from build123d import *

# Parameters (mm, degrees)
SKETCH1_R               = 15
BOSS_EXTRUDE1_DEPTH     = 27
SKETCH2_R               = 19.07
BOSS_EXTRUDE2_DEPTH     = 1.7
CUT_EXTRUDE1_DEPTH      = 23.4
SKETCH4_R               = 4
CUT_EXTRUDE2_DEPTH      = 5.3
SKETCH5_R               = 2.4
BOSS_EXTRUDE3_DEPTH     = 7
FILLET1_R               = 1
CUT_EXTRUDE3_DEPTH      = 44.397347845
CUT_EXTRUDE3_DEPTH_BACK = 44.397347845
SKETCH6_R               = 1.5


with BuildPart() as part:
    # Sketch1 → Boss-Extrude1 (new body)
    with BuildSketch(Plane(origin=(0, 0, 0), x_dir=(1, 0, 0), z_dir=(0, 1, 0))):
        with Locations(Location((0, 0, 0), (0, 0, 270))):
            Circle(SKETCH1_R)
    extrude(amount=BOSS_EXTRUDE1_DEPTH)

    # Sketch2 → Boss-Extrude2 (add)
    with BuildSketch(Plane.XZ):
        with Locations(Location((0, 0, 0), (0, 0, 270))):
            Circle(SKETCH2_R)
    extrude(amount=BOSS_EXTRUDE2_DEPTH)

    # Sketch3 → Cut-Extrude1 (cut)
    with BuildSketch(Plane.XZ.offset(1.7)):
        Polygon((-2.800148806, 4.85), (-5.600297611, 0), (-2.800148806, -4.85), (2.800148806, -4.85), (5.600297611, 0), (2.800148806, 4.85), align=None)
    extrude(amount=-CUT_EXTRUDE1_DEPTH, mode=Mode.SUBTRACT)

    # Sketch4 → Cut-Extrude2 (cut)
    with BuildSketch(Plane.XZ.offset(-21.7)):
        with Locations(Location((0, 0, 0), (0, 0, 270))):
            Circle(SKETCH4_R)
    extrude(amount=-CUT_EXTRUDE2_DEPTH, mode=Mode.SUBTRACT)

    # Sketch5 → Boss-Extrude3 (add)
    with BuildSketch(Plane(origin=(0, 27, 0), x_dir=(1, 0, 0), z_dir=(0, 1, 0))):
        with Locations(Location((-10, 0, 0), (0, 0, 270))):
            Circle(SKETCH5_R)
        with Locations(Location((10, 0, 0), (0, 0, 270))):
            Circle(SKETCH5_R)
    extrude(amount=BOSS_EXTRUDE3_DEPTH)

    # Fillet1
    fillet1_edges = [part.edges().sort_by_distance(p)[0] for p in [
        (-10, 34, -2.4),
        (10, 34, -2.4),
    ]]
    fillet(fillet1_edges, radius=FILLET1_R)

    # Sketch6 → Cut-Extrude3 (cut, two sides: drawn at the far end of the back side and taken through both)
    with BuildSketch(Plane.XY.offset(-CUT_EXTRUDE3_DEPTH_BACK)):
        with Locations(Location((0, 3, 0), (0, 0, 90))):
            Circle(SKETCH6_R)
    extrude(amount=CUT_EXTRUDE3_DEPTH + CUT_EXTRUDE3_DEPTH_BACK, mode=Mode.SUBTRACT)


solid = part.part
The listing builds one solid part. Answer for the finished solid, in the listing's coordinates (mm). A direction names the side the tool comes from. Coordinates: 2 decimals unless noted, no trailing zeros. Write each loop counter-clockwise with the first axis right and the second up, starting at its lowest first coordinate (ties: lowest second). Pieces come first, ordered by that corner, then holes. Notation, with made-up numbers: (67.5, -4) - (87.5, -4) arc R26 cw to (87.5, 28) - close; hole circle Ø11 at (-10.75, 29). An arc over 180 degrees is marked (long way). Answer as CSV lines item,"result".
1. Given P1, Ø10, axis at x = 13, y = 24, coming from the +Z side; P2, Ø3, axis at x = 0.5, y = 10, coming from the +Z side; P3, Ø8, axis at x = -8, y = 11.5, coming from the -Z side, each flat-ended and moving along its own axis, determine where each tip first touches the part or whether it passes through.
Computed values:
P1,"stops at z = 12.69"
P2,"stops at z = 15"
P3,"stops at z = -14.46"
2. A tool of negligible diameter and unlimited length cuts with its end or side. For faces 5 (the flat face through (-10, 34, 0)), 6 (the cylindrical face through (12.38, 29.96, -0.31)), 7 (the flat face through (0, 10, -4.85)), from which of +Z, -Z, +X, -X, +Y, -Y can it reach the whole face along a straight path? Write none if from no direction.
Computed values:
face 5,"+Z, -Z, +X, -X, +Y"
face 6,"+Y"
face 7,"-Y"
3. Find section B-B (x = 0). Give the vertices of the cut face in (y, z), plus the area to 3 significant figures.
Computed values:
outline,"(-1.7, -19.07) - (0, -19.07) - (0, -15) - (1.5, -15) - (1.5, -4.85) - (-1.7, -4.85) - close; (-1.7, 4.85) - (1.5, 4.85) - (1.5, 15) - (0, 15) - (0, 19.07) - (-1.7, 19.07) - close; (4.5, -15) - (27, -15) - (27, -4) - (21.7, -4) - (21.7, -4.85) - (4.5, -4.85) - close; (4.5, 4.85) - (21.7, 4.85) - (21.7, 4) - (27, 4) - (27, 15) - (4.5, 15) - close"
area,"545 mm²"
4. Straight lines are drawn through the part: line 1 (X direction, y = 23.05, z = 0); line 2 (Z direction, x = -0.5, y = 1); line 3 (Y direction, x = -12, z = -11). For each, find the intervals that lie inside material, in ascending order. Write a range as [from, to].
Computed values:
line 1,"x = [-15, -4], [4, 15]"
line 2,"z = [-14.99, -4.85], [4.85, 14.99]"
line 3,"y = [-1.7, 0]"
5. Find section C-C (y = 29). Give the vertices of the cut face in (x, z), plus the area to 3 significant figures.
Computed values:
outline,"circle Ø4.8 at (-10, 0); circle Ø4.8 at (10, 0)"
area,"36.2 mm²"
6. Find section A-A (y = 16.5). Give the vertices of the cut face in (x, z).
Computed values:
outline,"circle Ø30 at (0, 0); hole (-5.6, 0) - (-2.8, -4.85) - (2.8, -4.85) - (5.6, 0) - (2.8, 4.85) - (-2.8, 4.85) - close"
7. Find section D-D (z = -11). Give the vertices of the cut face in (x, y).
Computed values:
outline,"(-15.58, -1.7) - (15.58, -1.7) - (15.58, 0) - (10.2, 0) - (10.2, 27) - (-10.2, 27) - (-10.2, 0) - (-15.58, 0) - close; hole circle Ø3 at (0, 3)"
8. Determine the mould class of faces 1 (the cylindrical face through (-0.07, 1.5, 9.85)), 2 (the cylindrical face through (-0.07, 1.5, -10)), 3 (the cylindrical face through (-7.976, 29.958, 1.29)), 4 (the flat face through (-4, -1.7, -4)) for opening direction Y: +Y half, -Y half, draft (parallel to the pull), parting line (faces both ways), or undercut.
Computed values:
face 1,"undercut"
face 2,"undercut"
face 3,"draft"
face 4,"-Y half"
